from build123d import *

# Parameters (mm, degrees)
BOSS_EXTRUDE1_DEPTH = 6.35


with BuildPart() as part:
    # Sketch1 → Boss-Extrude1 (new body)
    with BuildSketch(Plane.XY):
        with BuildLine():
            Line((0, 2), (0, 8.7122))
            Line((0, 8.7122), (1.5748, 8.7122))
            Line((1.5748, 8.7122), (1.5748, 3.0748))
            ThreePointArc((1.5748, 3.0748), (2.014139828, 2.014139828), (3.0748, 1.5748))
            Line((3.0748, 1.5748), (9.525, 1.5748))
            Line((9.525, 1.5748), (9.525, 0))
            Line((9.525, 0), (2, 0))
            ThreePointArc((2, 0), (0.585786438, 0.585786438), (0, 2))
        make_face()
    extrude(amount=BOSS_EXTRUDE1_DEPTH)


solid = part.part
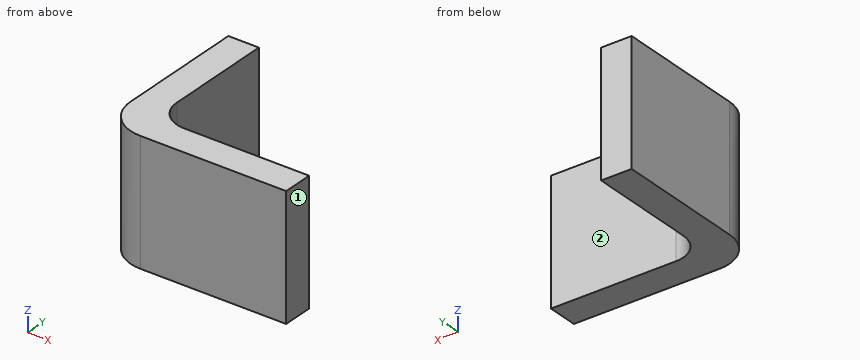
Could you check a few things on this model? Use its own coordinates, in mm. Face numbers are marked on the shaded views. A direction names the side the tool comes from. Give positions to 0.01 mm unless a question says otherwise; leave off trailing zeros. Order: outer loops, then holes, each group sorted by start corner. A loop starts at its lowest first (then second) coordinate and runs counter-clockwise, first axis right, second up. Notation, with made-up numbers: (21.25, -32.75) - (74.25, -32.75) arc R20 cw to (74.25, -0.75) - close; hole circle Ø9 at (-8, 78.5). An arc over 180 degrees is marked (long way). One line per question, with ' | ' between items. Start each with the question number.
Item 1: I'm going to push flat-ended pins straight in: pin 1 Ø3 at (x, z) = (6, 2.5) entering from +Y; pin 2 Ø5 at (x, y) = (8, 3.5) entering from -Z; pin 3 Ø1.5 at (y, z) = (5, 5) entering from +X. Where does each tip first touch, or does it pass through?
Item 2: I want a section at A-A on z = 5.75. Write out the boundary of the cut face in (x, y) (3 decimals).
Item 3: I need wall thicknesses on probe 1 along Y at (x, z) = (5.5, 5.5); probe 2 along Y at (x, z) = (2, 0.5). Which ranges of each line are inside material? Lowest first, please. Write a range as [from, to].
Item 4: For the marked faces 1 and 2, which set-ups out of +Z, -Z, +X, -X, +Y, -Y let a thin tool reach every point of the face, with its end or its side?
Item 5: I want a section at B-B on y = 6.5. Write out the boundary of the cut face in (x, z).
Verdict:
1) pin 1: y = 1.57 | pin 2: z = 0 | pin 3: x = 1.57
2) outline: (0, 2) arc R2 ccw to (2, 0) - (9.525, 0) - (9.525, 1.575) - (3.075, 1.575) arc R1.5 cw to (1.575, 3.075) - (1.575, 8.712) - (0, 8.712) - close
3) probe 1: [0, 1.57] | probe 2: [0, 2.03]
4) face 1: +Z, -Z, +X, +Y, -Y | face 2: +Z, -Z, +X, +Y
5) outline: (0, 0) - (1.57, 0) - (1.57, 6.35) - (0, 6.35) - close
